from build123d import *

# Parameters (mm, degrees)
SKETCH1_W           = 177.8
SKETCH1_H           = 25.4
BOSS_EXTRUDE1_DEPTH = 2.38125
SKETCH2_W           = 177.8
SKETCH2_H           = 25.4
BOSS_EXTRUDE2_DEPTH = 2.38125
FILLET1_R           = 2.38125


with BuildPart() as part:
    # Sketch1 → Boss-Extrude1 (new body)
    with BuildSketch(Plane(origin=(0, 0, 0), x_dir=(1, 0, 0), z_dir=(0, 1, 0))):
        with Locations((88.9, 12.7)):
            Rectangle(SKETCH1_W, SKETCH1_H)
    extrude(amount=BOSS_EXTRUDE1_DEPTH)

    # Sketch2 → Boss-Extrude2 (add)
    with BuildSketch(Plane.XY):
        with Locations((88.9, 12.7)):
            Rectangle(SKETCH2_W, SKETCH2_H)
    extrude(amount=BOSS_EXTRUDE2_DEPTH)

    # Fillet1
    fillet1_edges = [part.edges().sort_by_distance(p)[0] for p in [
        (88.9, 0, 2.38125),
    ]]
    fillet(fillet1_edges, radius=FILLET1_R)


solid = part.part
Read the model definition and answer for the solid it produces. Units are mm, in the model's axes. A direction names the side the tool comes from. Give positions to 0.01 mm unless a question says otherwise; leave off trailing zeros. Write each loop counter-clockwise with the first axis right and the second up, starting at its lowest first coordinate (ties: lowest second). Pieces come first, ordered by that corner, then holes. Notation, with made-up numbers: (50.5, -31.75) - (71.5, -31.75) arc R5 cw to (71.5, -26.75) - close; hole circle Ø4 at (88, 67). An arc over 180 degrees is marked (long way). Return JSON: item names as keys, results as strings.
Q1. Given P1, Ø4, axis at x = 76, y = 17.5, coming from the -Z side, flat-ended and moving along its own axis, determine where the tip first touches the part or whether it passes through.
Reply:
{"P1": "z = 0"}
Q2. For faces 1 (the face through (0, 2, -7)), 2 (the face through (88, 2.381, -13)), determine the directions among +Z, -Z, +X, -X, +Y, -Y from which every point of the face is accessible in a straight line to the end or side of a thin tool.
Reply:
{"face 1": "+Z, -Z, -X, +Y, -Y", "face 2": "-Z, +X, -X, +Y"}
Q3. A cutting plane is placed at A-A, the plane x = 56.5. Determine the outline of the cut face in (y, z).
Reply:
{"outline": "(0, -25.4) - (2.38, -25.4) - (2.38, 0) - (25.4, 0) - (25.4, 2.38) - (2.38, 2.38) arc R2.38 ccw to (0, 0) - close"}
Q4. A cutting plane is placed at B-B, the plane z = -21.25. Determine the outline of the cut face in (x, y).
Reply:
{"outline": "(0, 0) - (177.8, 0) - (177.8, 2.38) - (0, 2.38) - close"}
Q5. Consider line 1 along Y through (x, z) = (158, -13.75); line 2 along Y through (x, z) = (147.5, 1). Determine where each line is inside the solid, lowest interval first. Write a range as [from, to].
Reply:
{"line 1": "[0, 2.38]", "line 2": "[0.22, 25.4]"}
